Verification items for the finished model (mm, model axes). A direction names the side the tool comes from. Round coordinates to 2 decimals unless told otherwise and drop trailing zeros. Write each loop counter-clockwise with the first axis right and the second up, starting at its lowest first coordinate (ties: lowest second). Pieces come first, ordered by that corner, then holes. Notation, with made-up numbers: M 25,59.5 L 56,59.5 A34 ccw 56,95.5 Z; hole C 9,37.25 d5. An arc over 180 degrees is marked long. One line per item, written item: value. Start each with the question number.
Item 1: Tool access check on faces 1 (the face through (-7.5, 1, -1)), 2 (the face through (6.5, 10.6, -27.1)), 3 (the face through (1.3, 12.3, -34.5)). Record the directions out of +Z, -Z, +X, -X, +Y, -Y that give a thin tool (end or side, any length) a straight path to the whole face; none if there is none.
Item 2: Draft check along Y on faces 4 (the face through (0.228, 12.235, -36.021)), 5 (the face through (0.228, 1.479, 17.765)), 6 (the face through (0, 3, 0)). Enter one of: +Y half, -Y half, draft (parallel to the pull), parting line (faces both ways), or undercut.
Item 3: Section check A-A, the plane y = 14. Record the cut outline in (x, z), then the cut area to 3 significant figures.
Item 4: Gauge pin test, flat end, axial feed: pin 1 (3 mm diameter, centred on x = 1.5, z = -19, fed in from +Y). Record the tip position at first contact, or that the pin passes through.
Item 5: Thickness scan on probe 1 along Z at (x, y) = (0, 0.9); probe 2 along Z at (x, y) = (5.25, 12.5); probe 3 along Y at (x, z) = (2.25, -9.5). Record the ranges inside material, lowest first. Write a range as from..to.
Item 6: Section check D-D, the plane z = 32. Record the cut outline in (x, y).
Item 7: Section check B-B, the plane x = 0. Record the cut outline in (y, z).
Item 8: Section check C-C, the plane y = 10.5. Record the cut outline in (x, z).
Autodesk Inventor part; units mm, degrees
ref_plane "YZ Plane" through (0, 0, 0) normal (1, 0, 0) x (0, 1, 0)
ref_plane "XZ Plane" through (0, 0, 0) normal (0, 1, 0) x (-1, 0, 0)
ref_plane "XY Plane" through (0, 0, 0) normal (0, 0, 1) x (1, 0, 0)
sketch "Sketch1" plane through (0, 0, 0) normal (0, 1, 0) x (-1, 0, 0)
  line L0 (-7.5, 37.5) -> (7.5, 37.5)
  line L1 (7.5, 37.5) -> (7.5, -37.5)
  line L2 (7.5, -37.5) -> (-7.5, -37.5)
  line L3 (-7.5, -37.5) -> (-7.5, 37.5)
  line L4 (-7.5, 37.5) -> (7.5, -37.5) construction
  line L5 (7.5, 37.5) -> (-7.5, -37.5) construction
  circle A0 centre (0, 19.5) radius 1.75
  circle A1 centre (0, -19.5) radius 1.75
  point P0 (0, 0)
  point P1 (0, -37.5)
  dimension "d0" = 15
  dimension "d1" = 75
  dimension "d13" = 18
  dimension "d14" = 18
  dimension "d16" = 3.5
extrude "Extrusion1" add sketch "Sketch1" along normal blind 3
sketch "Sketch2" plane through (-7.5, 0, 37.5) normal (0, 0, 1) x (1, 0, 0)
  line L0 (0, 0) -> (15, 0)
  line L1 (15, 0) -> (15, 3)
  line L2 (0, 3) -> (15, 3)
  line L3 (0, 0) -> (0, 3)
  line L4 (15, 3) -> (0, 3)
  line L5 (0, 3) -> (15, 3)
  line L6 (15, 3) -> (15, 18)
  line L7 (15, 18) -> (0, 18)
  line L8 (0, 18) -> (0, 3)
  circle A0 centre (7.5, 10.5) radius 1.75
  point P0 (7.5, 0)
  point P1 (7.5, 18)
  point P2 (0, 10.5)
  dimension "d15" = 3.5
extrude "Extrusion2" add sketch "Sketch2" against normal blind 3 contours L8 L7 L6 L2
sketch "Sketch3" plane through (7.5, 0, -37.5) normal (0, 0, -1) x (-1, 0, 0)
  line L0 (15, 18) -> (0, 18)
  line L1 (0, 18) -> (0, 3)
  line L2 (15, 3) -> (0, 3)
  line L3 (15, 3) -> (15, 18)
  circle A0 centre (7.5, 10.5) radius 1.75
  point P0 (7.5, 0)
extrude "Extrusion3" add sketch "Sketch3" against normal blind 3
sketch "Sketch4" plane through (7.5, 0, 37.5) normal (1, 0, 0) x (0, 0, -1)
  line L0 (0, 0) -> (75, 0)
  line L1 (75, 0) -> (75, 18)
  line L2 (75, 18) -> (72, 18)
  line L3 (72, 3) -> (72, 18)
  line L4 (3, 3) -> (72, 3)
  line L5 (3, 18) -> (3, 3)
  line L6 (0, 18) -> (3, 18)
  line L7 (0, 0) -> (0, 18)
  line L8 (3, 18) -> (18, 3)
  line L9 (72, 3) -> (72, 18)
  line L10 (72, 18) -> (57, 3)
  line L11 (72, 3) -> (3, 3)
  point P0 (37.5, 0)
  dimension "d8" = 45
extrude "Extrusion4" add sketch "Sketch4" against normal blind 2 contours L8 L4 L5 | L3 L4 L10
sketch "Sketch5" plane through (-7.5, 0, -37.5) normal (-1, 0, 0) x (0, 0, 1)
  line L0 (18, 3) -> (3, 3)
  line L1 (18, 3) -> (3, 18)
  line L2 (3, 3) -> (3, 18)
  line L3 (72, 3) -> (57, 3)
  line L4 (72, 18) -> (72, 3)
  line L5 (72, 18) -> (57, 3)
  point P0 (37.5, 0)
extrude "Extrusion5" add sketch "Sketch5" against normal blind 2
equation "\"d14\" = d13"
properties part number "Frame_Brace_Mount" material "ABS Plastic"
Response values:
1. face 1: +Z, -Z, -X, +Y, -Y
1. face 2: +X, -X, +Y
1. face 3: +Y
2. face 4: undercut
2. face 5: draft
2. face 6: +Y half
3. outline: M -7.5,-37.5 L 7.5,-37.5 L 7.5,-30.5 L 5.5,-30.5 L 5.5,-34.5 L -5.5,-34.5 L -5.5,-30.5 L -7.5,-30.5 Z; M -7.5,30.5 L -5.5,30.5 L -5.5,34.5 L 5.5,34.5 L 5.5,30.5 L 7.5,30.5 L 7.5,37.5 L -7.5,37.5 Z
3. area: 122 mm2
4. pin 1: stops at y = 3
5. probe 1: z = -37.5..-21.25, -17.75..17.75, 21.25..37.5
5. probe 2: z = -37.5..-34.5, 34.5..37.5
5. probe 3: y = 0..3
6. outline: M -7.5,0 L 7.5,0 L 7.5,15.5 L 5.5,15.5 L 5.5,3 L -5.5,3 L -5.5,15.5 L -7.5,15.5 Z
7. outline: M 0,-37.5 L 8.75,-37.5 L 8.75,-34.5 L 3,-34.5 L 3,-21.25 L 0,-21.25 Z; M 0,-17.75 L 3,-17.75 L 3,17.75 L 0,17.75 Z; M 0,21.25 L 3,21.25 L 3,34.5 L 8.75,34.5 L 8.75,37.5 L 0,37.5 Z; M 12.25,-37.5 L 18,-37.5 L 18,-34.5 L 12.25,-34.5 Z; M 12.25,34.5 L 18,34.5 L 18,37.5 L 12.25,37.5 Z
8. outline: M -7.5,-37.5 L -1.75,-37.5 L -1.75,-34.5 L -5.5,-34.5 L -5.5,-27 L -7.5,-27 Z; M -7.5,27 L -5.5,27 L -5.5,34.5 L -1.75,34.5 L -1.75,37.5 L -7.5,37.5 Z; M 1.75,-37.5 L 7.5,-37.5 L 7.5,-27 L 5.5,-27 L 5.5,-34.5 L 1.75,-34.5 Z; M 1.75,34.5 L 5.5,34.5 L 5.5,27 L 7.5,27 L 7.5,37.5 L 1.75,37.5 Z
